The model under review builds one solid part; all positions refer to its coordinate system, in mm. A direction names the side the tool comes from. Round coordinates to 2 decimals unless told otherwise and drop trailing zeros. Write each loop counter-clockwise with the first axis right and the second up, starting at its lowest first coordinate (ties: lowest second). Pieces come first, ordered by that corner, then holes. Notation, with made-up numbers: (83, -31) -> (118, -31) arc R26 ccw to (118, -5) -> close; hole circle Ø6 at (-28.75, 46). An arc over 180 degrees is marked (long way). Return JSON: item names as keys, results as strings. Group by question number.
1. Tool access review of faces 1 (the cylindrical face through (-0.986, -1.734, -2.262)), 2 (the flat face through (15, 2, -1)): name each direction out of +Z, -Z, +X, -X, +Y, -Y from which nothing blocks a thin tool from reaching the whole face with its end or side.
2. Take a section at C-C, the plane y = -3.5. Give the number of separate pieces and of enclosed holes in the cut face, then the cut area to 3 significant figures.
3. Mouldability with a two-part tool opening along Z and no side actions: class faces 3 (the cylindrical face through (5, -2, 0)), 4 (the flat face through (0, 1, 3)), 5 (the conical face through (3.091, 0.987, -3.135)) as pulls with the +Z half, pulls with the -Z half, needs draft (parallel to the pull), parting line crosses it, or undercut.
4. For line 1 along Z through (x, y) = (-7.5, 1); line 2 along Y through (x, z) = (4.5, 1.25); line 3 along Y through (x, z) = (0.5, 0), list the stretches that pass through material, from the lowest coordinate up. Write a range as from..to.
5. Take a section at B-B, the plane x = 9. Write out the cut boundary in (y, z), then the cut area to 3 significant figures.
6. Clearance check with flat-ended pins moving along their axes: P1, Ø5, axis at x = 4.5, y = 2, coming from the -Z side; P2, Ø4, axis at x = -10.5, y = -3.5, coming from the -Z side; P3, Ø5, axis at x = -15, y = 3.5, coming from the -Z side. State where each tip first meets the part, or that it passes through.
from build123d import *

# Parameters (mm, degrees)
SKETCH1_R           = 4
BOSS_EXTRUDE1_DEPTH = 5
BOSS_EXTRUDE1_TAPER = 13
SKETCH2_R           = 4
BOSS_EXTRUDE2_DEPTH = 5
BOSS_EXTRUDE2_TAPER = 13
SKETCH3_R           = 4
BOSS_EXTRUDE3_DEPTH = 5
BOSS_EXTRUDE3_TAPER = 13
SKETCH4_R           = 2.85
BOSS_EXTRUDE4_DEPTH = 2
SKETCH5_R           = 2.85
BOSS_EXTRUDE5_DEPTH = 3
BOSS_EXTRUDE5_DRAFT = -35
SKETCH6_R           = 4.950622615
BOSS_EXTRUDE6_DEPTH = 15
BOSS_EXTRUDE6_TAPER = 12
SKETCH9_R           = 2
CUT_EXTRUDE1_DEPTH  = 20
SKETCH11_R          = 0.5
CUT_EXTRUDE2_DEPTH  = 15
CUT_EXTRUDE2_DRAFT  = 5.8


with BuildPart() as part:
    # Sketch1 → Boss-Extrude1 (new body)
    with BuildSketch(Plane(origin=(0, 0, 0), x_dir=(0, 0, -1), z_dir=(1, 0, 0))):
        Circle(SKETCH1_R)
    extrude(amount=BOSS_EXTRUDE1_DEPTH, taper=BOSS_EXTRUDE1_TAPER)

    # Sketch2 → Boss-Extrude2 (add)
    with BuildSketch(Plane(origin=(5, 0, 0), x_dir=(0, 0, -1), z_dir=(1, 0, 0))):
        Circle(SKETCH2_R)
    extrude(amount=BOSS_EXTRUDE2_DEPTH, taper=BOSS_EXTRUDE2_TAPER)

    # Sketch3 → Boss-Extrude3 (add)
    with BuildSketch(Plane(origin=(10, 0, 0), x_dir=(0, 0, -1), z_dir=(1, 0, 0))):
        Circle(SKETCH3_R)
    extrude(amount=BOSS_EXTRUDE3_DEPTH, taper=BOSS_EXTRUDE3_TAPER)

    # Sketch4 → Boss-Extrude4 (add)
    with BuildSketch(Plane.ZY):
        Circle(SKETCH4_R)
    extrude(amount=BOSS_EXTRUDE4_DEPTH)


with BuildPart() as boss_extrude5_tool:
    # Sketch5 → Boss-Extrude5 (with draft: the straight prism first)
    with BuildSketch(Plane.ZY.offset(2)):
        Circle(SKETCH5_R)
    extrude(amount=BOSS_EXTRUDE5_DEPTH)
    # Boss-Extrude5: the draft: its side faces are tilted about the plane it starts from
    boss_extrude5_sides = [boss_extrude5_tool.faces().sort_by_distance(p)[0] for p in [
        (-3.5, 0, -2.85),
    ]]
    draft(boss_extrude5_sides, Plane.ZY.offset(2), BOSS_EXTRUDE5_DRAFT)


with BuildPart() as part_1:
    add(part.part)

    # Boss-Extrude5: add boss_extrude5_tool
    add(boss_extrude5_tool.part)

    # Sketch6 → Boss-Extrude6 (add)
    with BuildSketch(Plane.ZY.offset(5)):
        Circle(SKETCH6_R)
    extrude(amount=BOSS_EXTRUDE6_DEPTH, taper=BOSS_EXTRUDE6_TAPER)

    # Sketch9 → Cut-Extrude1 (cut)
    with BuildSketch(Plane(origin=(15, 0, 0), x_dir=(0, 0, -1), z_dir=(1, 0, 0))):
        Circle(SKETCH9_R)
    extrude(amount=-CUT_EXTRUDE1_DEPTH, mode=Mode.SUBTRACT)


with BuildPart() as cut_extrude2_tool:
    # Sketch11 → Cut-Extrude2 (with draft: the straight prism first)
    with BuildSketch(Plane.ZY.offset(20)):
        Circle(SKETCH11_R)
    extrude(amount=-CUT_EXTRUDE2_DEPTH)
    # Cut-Extrude2: the draft: its side faces are tilted about the plane it starts from
    cut_extrude2_sides = [cut_extrude2_tool.faces().sort_by_distance(p)[0] for p in [
        (-12.5, 0, -0.5),
    ]]
    draft(cut_extrude2_sides, Plane.ZY.offset(20), CUT_EXTRUDE2_DRAFT)


with BuildPart() as part_2:
    add(part_1.part)

    # Cut-Extrude2: cut by cut_extrude2_tool
    add(cut_extrude2_tool.part, mode=Mode.SUBTRACT)


solid = part_2.part
Output:
{
 "1": {"face 1": "none", "face 2": "+Z, -Z, +X, +Y, -Y"},
 "2": {"separate pieces": "4", "enclosed holes": "0", "area": "56.6 mm^2"},
 "3": {"face 3": "undercut", "face 4": "needs draft", "face 5": "parting line crosses it"},
 "4": {"line 1": "z = -4.3..-1.46, 1.46..4.3", "line 2": "y = -2.68..-1.56, 1.56..2.68", "line 3": "y = -3.88..-2, 2..3.88"},
 "5": {"outline": "circle Ø6.15 at (0, 0); hole circle Ø4 at (0, 0)", "area": "17.2 mm^2"},
 "6": {"P1": "stops at z = -4", "P2": "stops at z = -3.58", "P3": "stops at z = -2.79"}
}
